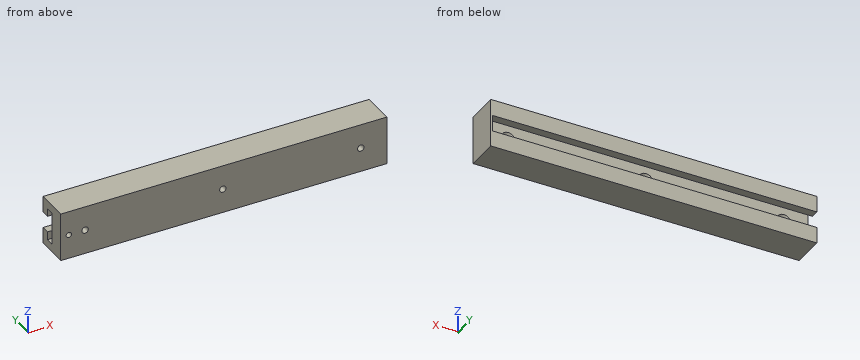
```python
from build123d import *

# Parameters (mm, degrees)
F0_W           = 5
F0_H           = 5
F1_DEPTH       = 200
F3_DEPTH       = 1.2
F5_D           = 4
F5_CSINK_D     = 8.7
F5_CSINK_ANGLE = 90
F6_DEPTH       = 25


with BuildPart() as f1:
    # F0 (on Right) → F1 (new body)
    with BuildSketch(Plane.YZ):
        Polygon((0, 30), (0, 15), (6.1031254008, 15), (10, 15), (10, 25), (15, 25), (20, 25), (20, 30), align=None)
        with Locations((17.5, 22.5)):
            Rectangle(F0_W, F0_H)
        with Locations((17.5, 7.5)):
            Rectangle(F0_W, F0_H)
        Polygon((0, 15), (0, 0), (20, 0), (20, 5), (15, 5), (10, 5), (10, 15), (6.1031254008, 15), align=None)
    extrude(amount=F1_DEPTH)

    # F2 (on face) → F3 (join)
    with BuildSketch(Plane.YZ.offset(200)):
        Polygon((20, 30), (0, 30), (0, 0), (20, 0), (20, 10), (15, 10), (15, 5), (10, 5), (10, 25), (15, 25), (15, 20), (20, 20), align=None)
        Polygon((20, 10), (20, 20), (15, 20), (15, 25), (10, 25), (10, 5), (15, 5), (15, 10), align=None)
    extrude(amount=F3_DEPTH)

    # F5 (through all)
    with Locations(Plane(origin=(0, 10, 0), x_dir=(-1, 0, 0), z_dir=(0, 1, 0))):
        with Locations((-15, 15), (-185, 15), (-100, 15)):
            CounterSinkHole(F5_D / 2, F5_CSINK_D / 2, counter_sink_angle=F5_CSINK_ANGLE)

    # F4 (on face) → F6 (cut)
    with BuildSketch(Plane(origin=(0, 10, 0), x_dir=(-1, 0, 0), z_dir=(0, 1, 0))):
        with BuildLine():
            ThreePointArc((-6.65, 15), (-5, 13.35), (-3.35, 15))
            Line((-3.35, 15), (-5, 15))
            Line((-5, 15), (-6.65, 15))
        make_face()
        with BuildLine():
            Line((-5, 15), (-3.35, 15))
            ThreePointArc((-3.35, 15), (-5, 16.65), (-6.65, 15))
            Line((-6.65, 15), (-5, 15))
        make_face()
    extrude(amount=-F6_DEPTH, mode=Mode.SUBTRACT)


solid = f1.part
```
Model file for the job. Use its own axes, mm. Coordinates: 2 decimals unless noted, no trailing zeros. Order: outer loops, then holes, each group sorted by start corner. A loop starts at its lowest first (then second) coordinate and runs counter-clockwise, first axis right, second up. Notation, with made-up numbers: (-33, 23) -> (-7, 23) arc R13 cw to (-7, 28) -> close; hole circle Ø6 at (14, -30). An arc over 180 degrees is marked (long way). Return JSON: item names as keys, results as strings.
Item 1: Slice it at C-C (x = 44). Write the cut outline in (y, z).
Model answer:
{"outline": "(0, 0) -> (20, 0) -> (20, 10) -> (15, 10) -> (15, 5) -> (10, 5) -> (10, 25) -> (15, 25) -> (15, 20) -> (20, 20) -> (20, 30) -> (0, 30) -> close"}
Item 2: Slice it at A-A (x = 5). Write the cut outline in (y, z), then the cut area to 3 significant figures.
Model answer:
{"outline": "(0, 0) -> (20, 0) -> (20, 10) -> (15, 10) -> (15, 5) -> (10, 5) -> (10, 13.35) -> (0, 13.35) -> close; (0, 16.65) -> (10, 16.65) -> (10, 25) -> (15, 25) -> (15, 20) -> (20, 20) -> (20, 30) -> (0, 30) -> close", "area": "417 mm²"}
Item 3: Pin check, flat tips, straight feed: P1, Ø3, axis at x = 15, z = 15, coming from the -Y side; P2, Ø5.5, axis at x = 5, z = 15, coming from the +Y side. Stop position of each tip, or through.
Model answer:
{"P1": "passes through", "P2": "stops at y = 10"}
Item 4: Wall check: line 1 along Z through (x, y) = (5, 3.25); line 2 along Z through (x, y) = (15, 5.5); line 3 along Y through (x, z) = (69, 8.25). Give the ranges that are in metal, low to high. Write a range as from..to.
Model answer:
{"line 1": "z = 0..13.35, 16.65..30", "line 2": "z = 0..13, 17..30", "line 3": "y = 0..10, 15..20"}
Item 5: Slice it at D-D (x = 100). Write the cut outline in (y, z), then the cut area to 3 significant figures.
Model answer:
{"outline": "(0, 0) -> (20, 0) -> (20, 10) -> (15, 10) -> (15, 5) -> (10, 5) -> (10, 10.65) -> (7.65, 13) -> (0, 13) -> close; (0, 17) -> (7.65, 17) -> (10, 19.35) -> (10, 25) -> (15, 25) -> (15, 20) -> (20, 20) -> (20, 30) -> (0, 30) -> close", "area": "404 mm²"}
Item 6: Slice it at B-B (z = 15). Write the cut outline in (x, y).
Model answer:
{"outline": "(0, 0) -> (3.35, 0) -> (3.35, 10) -> (0, 10) -> close; (6.65, 0) -> (13, 0) -> (13, 7.65) -> (10.65, 10) -> (6.65, 10) -> close; (17, 0) -> (98, 0) -> (98, 7.65) -> (95.65, 10) -> (19.35, 10) -> (17, 7.65) -> close; (102, 0) -> (183, 0) -> (183, 7.65) -> (180.65, 10) -> (104.35, 10) -> (102, 7.65) -> close; (187, 0) -> (201.2, 0) -> (201.2, 20) -> (200, 20) -> (200, 10) -> (189.35, 10) -> (187, 7.65) -> close"}
